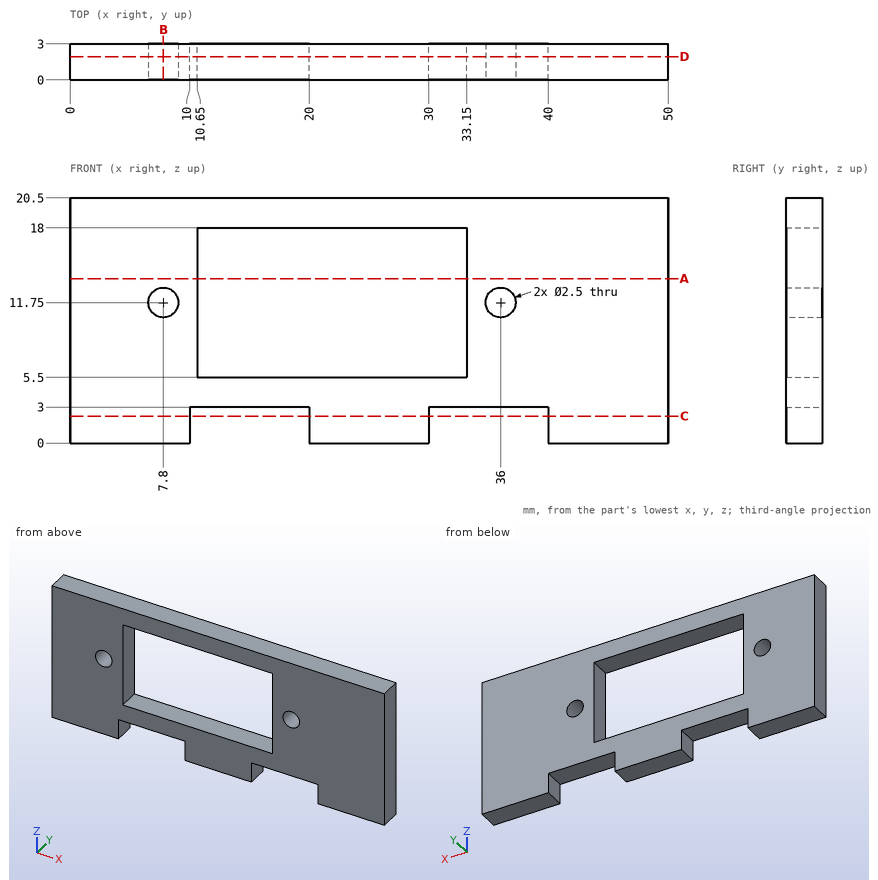
Study the drawing (mm; zero at the part's minimum x, y, z) and answer. Give positions to 0.01 mm unless a question says otherwise; leave off trailing zeros. Loops run counter-clockwise (first coordinate to the right, second up) from the corner with the lowest first, then second, coordinate; pieces in that order, holes last. Notation, with made-up numbers: (63.25, 50) -> (87.25, 50) arc R19 cw to (87.25, 83) -> close; hole circle Ø1 at (23.25, 85). An arc over 180 degrees is marked (long way). Use a Markdown table: item, result. Add a question column.
1) Each of these flat-tipped pins is pushed along its axis until it touches: P1, Ø2, axis at x = 7.8, z = 11.75, coming from the -Y side; P2, Ø0.9, axis at x = 34, y = 1, coming from the -Z side. Where does it stop, or does it pass through?
2) The part is cut by section B-B, the plane x = 7.8. Determine the outline of the cut face in (y, z).
3) The part is cut by section D-D, the plane y = 1.95. Determine the outline of the cut face in (x, z), plus the area to 3 significant figures.
4) The part is cut by section A-A, the plane z = 13.75. Determine the outline of the cut face in (x, y).
5) Consider line 1 along X through (y, z) = (1.8, 11.75); line 2 along X through (y, z) = (0.55, 15.75); line 3 along Z through (x, y) = (36, 2.15). Determine where each line is inside the solid, lowest interval first.
6) The part is cut by section C-C, the plane z = 2.25. Determine the outline of the cut face in (x, y).
Reported:
| question | item | result |
|---|---|---|
| 1 | P1 | passes through |
| 1 | P2 | stops at z = 3 |
| 2 | outline | (0, 0) -> (3, 0) -> (3, 10.5) -> (0, 10.5) -> close; (0, 13) -> (3, 13) -> (3, 20.5) -> (0, 20.5) -> close |
| 3 | outline | (0, 0) -> (10, 0) -> (10, 3) -> (20, 3) -> (20, 0) -> (30, 0) -> (30, 3) -> (40, 3) -> (40, 0) -> (50, 0) -> (50, 20.5) -> (0, 20.5) -> close; hole circle Ø2.5 at (7.8, 11.75); hole (10.65, 5.5) -> (33.15, 5.5) -> (33.15, 18) -> (10.65, 18) -> close; hole circle Ø2.5 at (36, 11.75) |
| 3 | area | 674 mm^2 |
| 4 | outline | (0, 0) -> (10.65, 0) -> (10.65, 3) -> (0, 3) -> close; (33.15, 0) -> (50, 0) -> (50, 3) -> (33.15, 3) -> close |
| 5 | line 1 | x = 0 to 6.55, 9.05 to 10.65, 33.15 to 34.75, 37.25 to 50 |
| 5 | line 2 | x = 0 to 10.65, 33.15 to 50 |
| 5 | line 3 | z = 3 to 10.5, 13 to 20.5 |
| 6 | outline | (0, 0) -> (10, 0) -> (10, 3) -> (0, 3) -> close; (20, 0) -> (30, 0) -> (30, 3) -> (20, 3) -> close; (40, 0) -> (50, 0) -> (50, 3) -> (40, 3) -> close |
